Here's how the part is built. I have some questions about the finished solid (model axes, mm). Face numbers are marked on the shaded views. A direction names the side the tool comes from. Give positions to 0.01 mm unless a question says otherwise; leave off trailing zeros. Write each loop counter-clockwise with the first axis right and the second up, starting at its lowest first coordinate (ties: lowest second). Pieces come first, ordered by that corner, then holes. Notation, with made-up numbers: (68.5, 15) - (73.5, 15) arc R5 ccw to (73.5, 21) - close; hole circle Ø10 at (49, -1.5). An arc over 180 degrees is marked (long way). Use a Markdown table: item, result.
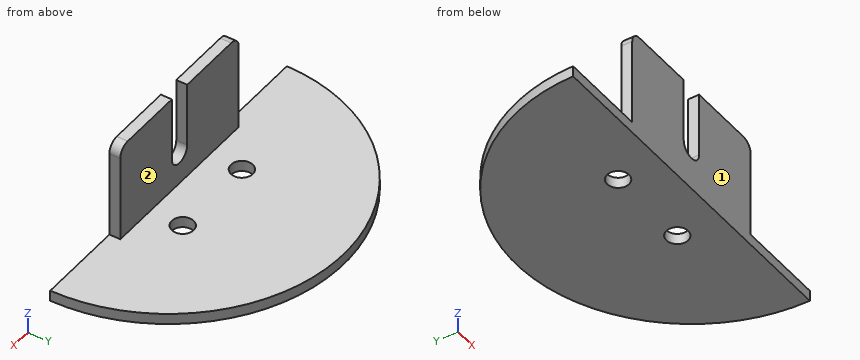
Autodesk Inventor part; units mm, degrees
ref_plane "YZ Plane" through (0, 0, 0) normal (1, 0, 0) x (0, 1, 0)
ref_plane "XZ Plane" through (0, 0, 0) normal (0, 1, 0) x (-1, 0, 0)
ref_plane "XY Plane" through (0, 0, 0) normal (0, 0, 1) x (1, 0, 0)
sketch "Sketch1" plane through (0, 0, 0) normal (0, 0, 1) x (1, 0, 0)
  arc A0 (50.8, 0) -> (-50.8, 0) centre (0, 0) ccw
  line L0 (0, 0) -> (50.8, 0)
  line L1 (0, 0) -> (-50.8, 0)
  dimension "d0" = 101.6
extrude "Extrusion1" add sketch "Sketch1" along normal blind 3.175
sketch "Sketch2" plane through (0, 0, 3.175) normal (0, 0, 1) x (1, 0, 0)
  arc A0 (50.8, 0) -> (-50.8, 0) centre (0, 0) ccw
  arc A1 (50.8, 0) -> (-50.8, 0) centre (0, 0) ccw
  line L0 (-50.8, 0) -> (50.8, 0)
  line L1 (0, 3.175) -> (0, 0) construction
  line L2 (0, 3.175) -> (25.4, 3.175)
  line L3 (25.4, 3.175) -> (25.4, 0)
  line L4 (-50.8, 0) -> (50.8, 0)
  line L5 (0, 3.175) -> (-25.4, 3.175)
  line L6 (-25.4, 3.175) -> (-25.4, 0)
  dimension "d6" = 25.4
  dimension "d7" = 3.175
extrude "Extrusion2" add sketch "Sketch2" along normal blind 28.575 contours L0 L6 L5 L2 L3
fillet "Fillet1" radius 3.175 2 edges at (25.4, 1.5875, 31.75) (-25.4, 1.5875, 31.75)
sketch "Sketch3" plane through (-25.4, 3.175, 3.175) normal (0, 1, 0) x (1, 0, 0)
  line L0 (25.4, 3.175) -> (25.4, -28.575) construction
  line L1 (3.175, -28.575) -> (47.625, -28.575) construction
  line L2 (25.4, -28.575) -> (25.4, -6.35) construction
  line L3 (22.098, -25.273) -> (22.098, -9.652)
  line L4 (28.702, -9.652) -> (28.702, -25.273)
  arc A0 (22.098, -25.273) -> (28.702, -25.273) centre (25.4, -25.273) ccw
  arc A1 (28.702, -9.652) -> (22.098, -9.652) centre (25.4, -9.652) ccw
  line L5 (0, 0) -> (50.8, 0)
  line L6 (22.098, -25.273) -> (22.098, -28.575)
  line L7 (28.702, -25.273) -> (28.702, -28.575)
  line L8 (22.098, -28.575) -> (28.702, -28.575)
  point P0 (25.4, -17.4625)
  dimension "d11" = 6.35
  dimension "d12" = 6.604
extrude "Extrusion3" cut sketch "Sketch3" against normal up to surface (3.175 mm away)
sketch "Sketch4" plane through (0, 0, 0) normal (0, 0, -1) x (-1, 0, 0)
  line L0 (0, 0) -> (0, 12.7) construction
  line L1 (0, 12.7) -> (12.7, 12.7) construction
  circle A0 centre (12.7, 12.7) radius 3.175
  circle A1 centre (-12.7, 12.7) radius 3.175
  dimension "d15" = 12.7
  dimension "d16" = 12.7
  dimension "d17" = 6.35
extrude "Extrusion4" cut sketch "Sketch4" against normal up to surface (3.175 mm away)
properties part number "Front with Plate"
Item 1: For the marked faces 1 and 2, which set-ups out of +Z, -Z, +X, -X, +Y, -Y let a thin tool reach every point of the face, with its end or its side?
Values:
| item | result |
|---|---|
| face 1 | +Z, -Z, +X, -X, -Y |
| face 2 | +Z, +X, -X, +Y |
Item 2: If we section it at A-A, the plane z = 17: Write out the boundary of the cut face in (x, y) (3 decimals), plus the area to 3 significant figures.
Values:
| item | result |
|---|---|
| outline | (-25.4, 0) - (-3.302, 0) - (-3.302, 3.175) - (-25.4, 3.175) - close; (3.302, 0) - (25.4, 0) - (25.4, 3.175) - (3.302, 3.175) - close |
| area | 140 mm2 |
Item 3: If we section it at B-B, the plane x = 12.7: Write out the boundary of the cut face in (y, z) (3 decimals), plus the area to 3 significant figures.
Values:
| item | result |
|---|---|
| outline | (0, 0) - (9.525, 0) - (9.525, 3.175) - (3.175, 3.175) - (3.175, 31.75) - (0, 31.75) - close; (15.875, 0) - (49.187, 0) - (49.187, 3.175) - (15.875, 3.175) - close |
| area | 227 mm2 |
Item 4: Will these pins go through, and if not, where does the flat tip stop? pin 1 Ø1 at (y, z) = (1.5, 21.5) entering from +X; pin 2 Ø3.5 at (y, z) = (1, 19.5) entering from -X; pin 3 Ø8 at (x, z) = (7.5, 4.5) entering from +Y; pin 4 Ø12 at (y, z) = (19.5, 10.5) entering from +X.
Values:
| item | result |
|---|---|
| pin 1 | stops at x = 25.4 |
| pin 2 | stops at x = -25.4 |
| pin 3 | stops at y = 50.66 |
| pin 4 | passes through |
Item 5: If we section it at D-D, the plane z = 5.5: Write out the boundary of the cut face in (x, y) (3 decimals), plus the area to 3 significant figures.
Values:
| item | result |
|---|---|
| outline | (-25.4, 0) - (25.4, 0) - (25.4, 3.175) - (-25.4, 3.175) - close |
| area | 161 mm2 |
Item 6: If we section it at C-C, the plane y = 12.7: Write out the boundary of the cut face in (x, z) (3 decimals), plus the area to 3 significant figures.
Values:
| item | result |
|---|---|
| outline | (-49.187, 0) - (-15.875, 0) - (-15.875, 3.175) - (-49.187, 3.175) - close; (-9.525, 0) - (9.525, 0) - (9.525, 3.175) - (-9.525, 3.175) - close; (15.875, 0) - (49.187, 0) - (49.187, 3.175) - (15.875, 3.175) - close |
| area | 272 mm2 |
Item 7: I need wall thicknesses on line 1 along X through (y, z) = (2, 24); line 2 along X through (y, z) = (12, 1); line 3 along Z through (x, y) = (38.5, 12) (3 decimals). Which ranges of each line are inside material? Lowest first, please. Write a range as [from, to].
Values:
| item | result |
|---|---|
| line 1 | x = [-25.4, -3.3], [3.3, 25.4] |
| line 2 | x = [-49.36, -15.8], [-9.6, 9.6], [15.8, 49.36] |
| line 3 | z = [0, 3.175] |
